from build123d import *

# Parameters (mm, degrees)
F0_W          = 50.8
F0_H          = 355.6
F0_R          = 12.7
F1_DEPTH      = 101.6
F1_DEPTH_BACK = 101.6
F2_W          = 101.6
F2_H          = 305.054
F3_DEPTH      = 38.1
F4_R          = 9.525
F5_DEPTH      = 101.6


with BuildPart() as f1:
    # F0 (on Right) → F1 (new body, two sides)
    with BuildSketch(Plane.YZ) as f1_sk:
        with Locations((0, 127.68995)):
            Rectangle(F0_W, F0_H)
        with Locations((0, -19.287717)):
            Circle(F0_R, mode=Mode.SUBTRACT)
    extrude(amount=F1_DEPTH)
    extrude(f1_sk.sketch, amount=-F1_DEPTH_BACK)

    # F2 (on face) → F3 (cut)
    with BuildSketch(Plane(origin=(0, 25.4, 0), x_dir=(-1, 0, 0), z_dir=(0, 1, 0))):
        with Locations((0, 146.61295)):
            Rectangle(F2_W, F2_H)
    extrude(amount=-F3_DEPTH, mode=Mode.SUBTRACT)

    # F4 (on face) → F5 (join, through all)
    with BuildSketch(Plane.YZ.offset(-50.8)):
        with Locations((6.35, 276.91495)):
            Circle(F4_R)
    extrude(amount=F5_DEPTH)


solid = f1.part
Geometry: final body of the model. Coordinates: model frame, mm. A direction names the side the tool comes from. Coordinates: 2 decimals unless noted, no trailing zeros. Write each loop counter-clockwise with the first axis right and the second up, starting at its lowest first coordinate (ties: lowest second). Pieces come first, ordered by that corner, then holes. Notation, with made-up numbers: (75, -16) - (133, -16) arc R31 cw to (133, 14) - close; hole circle Ø11 at (59, 31). An arc over 180 degrees is marked (long way). Return JSON: item names as keys, results as strings.
Item 1: Section query C-C (z = 22). Output: boundary loops of the cut face in (x, y), and give its area (3 significant figures).
Completed:
{"outline": "(-101.6, -25.4) - (101.6, -25.4) - (101.6, 25.4) - (50.8, 25.4) - (50.8, -12.7) - (-50.8, -12.7) - (-50.8, 25.4) - (-101.6, 25.4) - close", "area": "6,450 mm2"}
Item 2: Reachability of faces 1 (the face through (101.6, 0, 130)), 2 (the face through (1, 7, 299.14)), 3 (the face through (-0.71, 5.11, 286.36)) from +Z, -Z, +X, -X, +Y, -Y: full face, straight path, thin tool, end or side. Return the list, or none.
Completed:
{"face 1": "+Z, -Z, +X, +Y, -Y", "face 2": "+Y", "face 3": "none"}
Item 3: Pull-direction query (Z, two-part tool) for faces 4 (the face through (-101.6, 0, 130)), 5 (the face through (1, 0, -50.11)), 6 (the face through (1, 7, -5.914)); classes: +Z half, -Z half, draft (parallel to the pull), parting line (faces both ways), or undercut.
Completed:
{"face 4": "draft", "face 5": "-Z half", "face 6": "undercut"}
Item 4: Section query B-B (x = -32). Output: boundary loops of the cut face in (y, z) (3 decimals), and give its area (3 significant figures).
Completed:
{"outline": "(-25.4, -50.11) - (25.4, -50.11) - (25.4, -5.914) - (-12.7, -5.914) - (-12.7, 299.14) - (25.4, 299.14) - (25.4, 305.49) - (-25.4, 305.49) - close; circle Ø19.05 at (6.35, 276.915); hole circle Ø25.4 at (0, -19.288)", "area": "6,220 mm2"}
Item 5: Pin query (flat end, axial travel): pin 1 Ø2 at (x, z) = (22, 25) entering from +Y. Return the tip coordinate at first contact, or that it passes through.
Completed:
{"pin 1": "stops at y = -12.7"}
Item 6: Section query A-A (y = 6.35). Output: boundary loops of the cut face in (x, z), and give its area (3 significant figures).
Completed:
{"outline": "(-101.6, -50.11) - (101.6, -50.11) - (101.6, -30.29) - (-101.6, -30.29) - close; (-101.6, -8.29) - (101.6, -8.29) - (101.6, 305.49) - (-101.6, 305.49) - close; hole (-50.8, -5.91) - (50.8, -5.91) - (50.8, 267.39) - (-50.8, 267.39) - close; hole (-50.8, 286.44) - (50.8, 286.44) - (50.8, 299.14) - (-50.8, 299.14) - close", "area": "38,700 mm2"}
Item 7: Line query: L1, parallel to X at y = 15.5, z = 254.5; L2, parallel to Z at x = 61, y = 0; L3, parallel to Z at x = 30.5, y = 22.5. Output: solid intervals per line, ascending.
Completed:
{"L1": "x = -101.6 to -50.8, 50.8 to 101.6", "L2": "z = -50.11 to -31.99, -6.59 to 305.49", "L3": "z = -50.11 to -5.91, 299.14 to 305.49"}
Item 8: Section query D-D (x = 69). Output: boundary loops of the cut face in (y, z), and give its area (3 significant figures).
Completed:
{"outline": "(-25.4, -50.11) - (25.4, -50.11) - (25.4, 305.49) - (-25.4, 305.49) - close; hole circle Ø25.4 at (0, -19.29)", "area": "17,600 mm2"}
